```python
from build123d import *

# Parameters (mm, degrees)
SCHNITT_LINEAR_START                    = -20
SCHNITT_LINEAR_AUSTRAGEN1_OUTLINE_R     = 4.5
SCHNITT_LINEAR_AUSTRAGEN1_OUTLINE_R_2   = 2
SCHNITT_LINEAR_AUSTRAGEN1_DEPTH         = 6.199999898
SCHNITT_LINEAR_START_2                  = -12.199999898
SCHNITT_LINEAR_AUSTRAGEN1_2_OUTLINE_R   = 4.5
SCHNITT_LINEAR_AUSTRAGEN1_2_OUTLINE_R_2 = 2
SCHNITT_LINEAR_AUSTRAGEN1_2_DEPTH       = 6.199999898
SCHNITT_LINEAR_START_3                  = 6.199999898
SCHNITT_LINEAR_AUSTRAGEN1_3_OUTLINE_R   = 4.5
SCHNITT_LINEAR_AUSTRAGEN1_3_OUTLINE_R_2 = 2
SCHNITT_LINEAR_AUSTRAGEN1_3_DEPTH       = 1.600000204
SCHNITT_LINEAR_START_4                  = 1
SCHNITT_LINEAR_AUSTRAGEN1_4_OUTLINE_R   = 0.8
SCHNITT_LINEAR_AUSTRAGEN1_4_DEPTH       = 5
SKIZZE5_R                               = 0.85
SCHNITT_LINEAR_AUSTRAGEN2_DEPTH         = 30
SCHNITT_LINEAR_START_5                  = -4.5
SKIZZE6_R                               = 4.5
SCHNITT_LINEAR_AUSTRAGEN3_DEPTH         = 4.5
FASE1_SIZE                              = 0.3


with BuildPart() as part:
    # Schnitt-Linear austragen1: read off the stored shape, not the designer's step
    # Schnitt-Linear austragen1 outline → Schnitt-Linear austragen1 (new body)
    with BuildSketch(Plane(origin=(20, 0, 0), x_dir=(0, 0, -1), z_dir=(1, 0, 0)).offset(SCHNITT_LINEAR_START)):
        Circle(SCHNITT_LINEAR_AUSTRAGEN1_OUTLINE_R)
        Circle(SCHNITT_LINEAR_AUSTRAGEN1_OUTLINE_R_2, mode=Mode.SUBTRACT)
    extrude(amount=SCHNITT_LINEAR_AUSTRAGEN1_DEPTH)



with BuildPart() as body_2:
    # Schnitt-Linear austragen1 2 outline → Schnitt-Linear austragen1 2 (new body)
    with BuildSketch(Plane(origin=(20, 0, 0), x_dir=(0, 0, -1), z_dir=(1, 0, 0)).offset(SCHNITT_LINEAR_START_2)):
        Circle(SCHNITT_LINEAR_AUSTRAGEN1_2_OUTLINE_R)
        Circle(SCHNITT_LINEAR_AUSTRAGEN1_2_OUTLINE_R_2, mode=Mode.SUBTRACT)
    extrude(amount=SCHNITT_LINEAR_AUSTRAGEN1_2_DEPTH)


with BuildPart() as part_1:
    add(part.part)

    add(body_2.part)  # Schnitt-Linear austragen1 3 merges body 2
    # Schnitt-Linear austragen1 3 outline → Schnitt-Linear austragen1 3 (add)
    with BuildSketch(Plane.YZ.offset(SCHNITT_LINEAR_START_3)):
        Circle(SCHNITT_LINEAR_AUSTRAGEN1_3_OUTLINE_R)
        Circle(SCHNITT_LINEAR_AUSTRAGEN1_3_OUTLINE_R_2, mode=Mode.SUBTRACT)
    extrude(amount=SCHNITT_LINEAR_AUSTRAGEN1_3_DEPTH)

    # Schnitt-Linear austragen1 4 outline → Schnitt-Linear austragen1 4 (cut)
    with BuildSketch(Plane.XY.offset(SCHNITT_LINEAR_START_4)):
        with Locations((7, 0)):
            Circle(SCHNITT_LINEAR_AUSTRAGEN1_4_OUTLINE_R)
    extrude(amount=SCHNITT_LINEAR_AUSTRAGEN1_4_DEPTH, mode=Mode.SUBTRACT)

    # Skizze4 → Rotation1 (revolve)
    with BuildSketch(Plane(origin=(0, 0, 0), x_dir=(1, 0, 0), z_dir=(0, 1, 0))):
        Polygon((4.5, -4), (4.5, -12.25), (5.5, -12.25), (5.5, -9.25), (8.5, -9.25), (8.5, -12.25), (9.5, -12.25), (9.5, -4), align=None)
    revolve(axis=Axis((2.33899179, 0, 0), (1, 0, 0)))

    # Skizze5 → Schnitt-Linear austragen2 (cut)
    with BuildSketch(Plane.XY):
        with Locations(Location((7, 0, 0), (0, 0, 180))):
            Circle(SKIZZE5_R)
    extrude(amount=SCHNITT_LINEAR_AUSTRAGEN2_DEPTH, mode=Mode.SUBTRACT)

    # Skizze6 → Schnitt-Linear austragen3 (cut)
    with BuildSketch(Plane(origin=(14, 0, 0), x_dir=(0, 0, -1), z_dir=(1, 0, 0)).offset(SCHNITT_LINEAR_START_5)):
        with Locations(Location((0, 0, 0), (0, 0, 180))):
            Circle(SKIZZE6_R)
    extrude(amount=SCHNITT_LINEAR_AUSTRAGEN3_DEPTH, mode=Mode.SUBTRACT)

    # Fase1
    # the kernel refuses this chamfer: 0.3 mm, written as the material it takes off along each edge
    with BuildSketch(Plane(origin=(4.5, 0, 0), x_dir=(0, 0, 1), z_dir=(0, 1, 0))) as fase1_piece_1:
        Polygon((12.25 - FASE1_SIZE, 0), (12.25, FASE1_SIZE), (12.25, 0), align=None)
    revolve(axis=Axis((4.5, 0, 0), (1, 0, 0)), mode=Mode.SUBTRACT)
    with BuildSketch(Plane(origin=(5.5, 0, 0), x_dir=(0, 0, 1), z_dir=(0, 1, 0))) as fase1_piece_2:
        Polygon((12.25, -FASE1_SIZE), (12.25 - FASE1_SIZE, 0), (12.25, 0), align=None)
    revolve(axis=Axis((5.5, 0, 0), (1, 0, 0)), mode=Mode.SUBTRACT)
    with BuildSketch(Plane(origin=(8.5, 0, 0), x_dir=(0, 0, 1), z_dir=(0, 1, 0))) as fase1_piece_3:
        Polygon((12.25 - FASE1_SIZE, 0), (12.25, FASE1_SIZE), (12.25, 0), align=None)
    revolve(axis=Axis((8.5, 0, 0), (1, 0, 0)), mode=Mode.SUBTRACT)
    with BuildSketch(Plane(origin=(9.5, 0, 0), x_dir=(0, 0, 1), z_dir=(0, 1, 0))) as fase1_piece_4:
        Polygon((12.25, -FASE1_SIZE), (12.25 - FASE1_SIZE, 0), (12.25, 0), align=None)
    revolve(axis=Axis((9.5, 0, 0), (1, 0, 0)), mode=Mode.SUBTRACT)
    with BuildSketch(Plane(origin=(9.5, 0, 0), x_dir=(0, 0, -1), z_dir=(0, -1, 0))) as fase1_piece_5:
        Polygon((2 + FASE1_SIZE, 0), (2, -FASE1_SIZE), (2, 0), align=None)
    revolve(axis=Axis((9.5, 0, 0), (1, 0, 0)), mode=Mode.SUBTRACT)
    with BuildSketch(Plane(origin=(0, 0, 0), x_dir=(0, 0, -1), z_dir=(0, -1, 0))) as fase1_piece_6:
        Polygon((2, FASE1_SIZE), (2 + FASE1_SIZE, 0), (2, 0), align=None)
    revolve(axis=Axis((0, 0, 0), (1, 0, 0)), mode=Mode.SUBTRACT)
    with BuildSketch(Plane(origin=(0, 0, 0), x_dir=(0, 0, -1), z_dir=(0, -1, 0))) as fase1_piece_7:
        Polygon((4.5, FASE1_SIZE), (4.5 - FASE1_SIZE, 0), (4.5, 0), align=None)
    revolve(axis=Axis((0, 0, 0), (1, 0, 0)), mode=Mode.SUBTRACT)


solid = part_1.part
```
Build history of the part. All positions in model axes, mm. A direction names the side the tool comes from. Round coordinates to 2 decimals unless told otherwise and drop trailing zeros. Write each loop counter-clockwise with the first axis right and the second up, starting at its lowest first coordinate (ties: lowest second). Pieces come first, ordered by that corner, then holes.
1) Band-saw the part on B-B, the plane y = 0. Give the number of separate pieces and of enclosed holes in the cut face, and give its area (3 significant figures).
2) Mould opens along Y. For faces 1 (the cylindrical face through (7.02, 9.03, -2.01)), 2 (the cylindrical face through (6.215, 0.326, 5.478)), 3 (the flat face through (9.5, 2.5, -0.2)), 4 (the cylindrical face through (4.69, 0.74, -1.86)) say: +Y half, -Y half, draft (parallel to the pull), parting line (faces both ways), or undercut.
3) Band-saw the part on D-D, the plane x = 7. List the corners of the cut face in (y, z), and give its area (3 significant figures).
4) 3-axis set-ups, long thin cutter, end or side, ignore diameter. For faces 5 (the flat face through (8.5, 9, -3)), 6 (the flat face through (4.5, 0, -5)), 7 (the cylindrical face through (5.003, -10.329, 6.586)): which of +Z, -Z, +X, -X, +Y, -Y reach the whole face in a straight line?
5) Drill centre lines: probe 1 along X at (y, z) = (4.25, 8.5); probe 2 along Y at (x, z) = (7, 4.25); probe 3 along Y at (x, z) = (7, 6.5). Where is each one in solid material? Low to high.
6) Pin check, flat tips, straight feed: pin 1 (1 mm diameter, centred on x = 7, y = 0.5, fed in from -Z); pin 2 (1 mm diameter, centred on x = 5, y = -3, fed in from +Z); pin 3 (1.5 mm diameter, centred on x = 4.5, z = 2, fed in from -Y). Stop position of each tip, or through.
7) Band-saw the part on C-C, the plane x = 2. List the corners of the cut face in (y, z).
Ans:
1. separate pieces: 3
1. enclosed holes: 0
1. area: 94.0 mm2
2. face 1: parting line
2. face 2: undercut
2. face 3: draft
2. face 4: undercut
3. outline: (-0.85, 1.81) - (-0.85, 9.21) arc R9.25 ccw (long way) to (0.85, 9.21) - (0.85, 1.81) arc R2 cw (long way) to start
3. area: 244 mm2
4. face 5: none
4. face 6: -X
4. face 7: +X, -X
5. probe 1: x = 4.5 to 5.5, 8.5 to 9.5
5. probe 2: y = -8.22 to -0.85, 0.85 to 8.22
5. probe 3: y = -6.58 to -0.85, 0.85 to 6.58
6. pin 1: stops at z = -9.25
6. pin 2: stops at z = 11.99
6. pin 3: stops at y = -12.18
7. outline: circle Ø9 at (0, 0); hole circle Ø4 at (0, 0)
